Job drawing, mm, ordinate dimensions from the low corner. One solid piece. A direction names the side the tool comes from. Coordinates: 2 decimals unless noted, no trailing zeros. Loops run counter-clockwise (first coordinate to the right, second up) from the corner with the lowest first, then second, coordinate; pieces in that order, holes last. Notation, with made-up numbers: (-6, -36) -> (14, -36) arc R37 cw to (14, 1) -> close; hole circle Ø2 at (0.5, -8.5). An arc over 180 degrees is marked (long way). Use one line per item in the form item = value. Start each with the question number.
(1) Mould opens along X. For the marked faces 5, 6 and 7 say: +X half, -X half, draft (parallel to the pull), parting line (faces both ways), or undercut.
(2) Drill centre lines: L1, parallel to Y at x = 47, z = 21; L2, parallel to Z at x = 23.5, y = 39.5; L3, parallel to Y at x = 7, z = 11 (1 decimal). Where is each one in solid material? Low to high. Write a range as [from, to].
(3) Band-saw the part on D-D on x = 19. Give the cut face in (y, z).
(4) Pin check, flat tips, straight feed: P1, Ø10, axis at x = 13, y = 72, coming from the +Z side; P2, Ø14, axis at y = 19.5, z = 5.5, coming from the -X side; P3, Ø1.5, axis at x = 16, z = 28, coming from the +Y side. Stop position of each tip, or through.
(5) Band-saw the part on C-C on y = 10. Give the cut face in (x, z) (1 decimal).
(6) 3-axis set-ups, long thin cutter, end or side, ignore diameter. For the marked faces 1, 2, 3 and 4: which of +Z, -Z, +X, -X, +Y, -Y reach the whole face in a straight line?
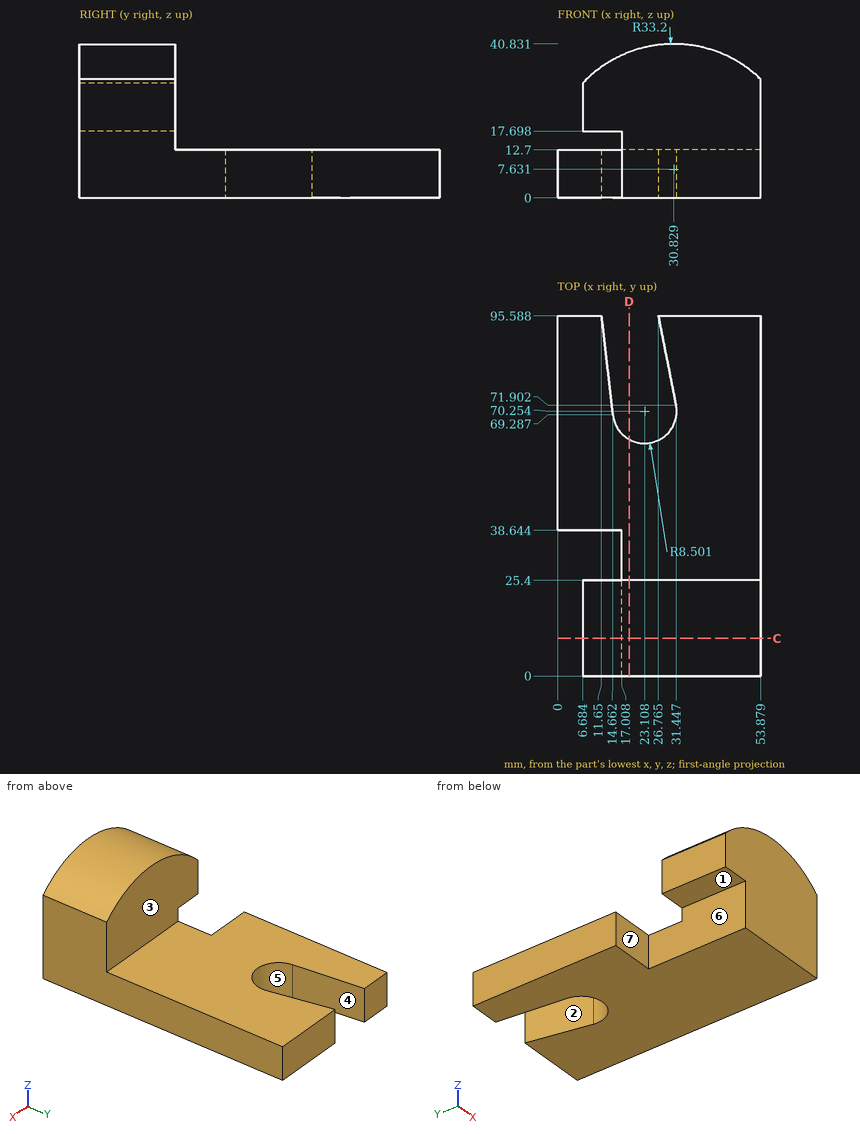
A:
q1.face_5 = undercut
q1.face_6 = -X half
q1.face_7 = draft
q2.L1 = [0, 25.4]
q2.L2 = [0, 12.7]
q2.L3 = [38.6, 95.6]
q3.outline = (0, 0) -> (62.81, 0) -> (62.81, 12.7) -> (25.4, 12.7) -> (25.4, 38.65) -> (0, 38.65) -> close
q4.P1 = 12.7
q4.P2 = 17.01
q4.P3 = 25.4
q5.outline = (6.7, 17.7) -> (17, 17.7) -> (17, 0) -> (53.9, 0) -> (53.9, 31.5) arc R33.2 ccw to (6.7, 30.4) -> close
q6.face_1 = -Z, -X, +Y, -Y
q6.face_2 = +Z, -Z
q6.face_3 = +Z, +X, -X, +Y
q6.face_4 = +Z, -Z, +Y
